Autodesk Inventor part; units mm, degrees
ref_plane "YZ Plane" through (0, 0, 0) normal (1, 0, 0) x (0, 1, 0)
ref_plane "XZ Plane" through (0, 0, 0) normal (0, 1, 0) x (-1, 0, 0)
ref_plane "XY Plane" through (0, 0, 0) normal (0, 0, 1) x (1, 0, 0)
sketch "Sketch1" plane through (0, 0, 0) normal (0, 0, 1) x (1, 0, 0)
  point P0 (0, 0)
sketch "Sketch2" plane through (0, 0, 0) normal (0, 0, 1) x (1, 0, 0)
  line L0 (-15, 20) -> (15, 20)
  line L1 (15, 20) -> (15, 0)
  line L2 (15, 0) -> (-15, 0)
  line L3 (-15, 0) -> (-15, 20)
  point P0 (0, 0)
  dimension "d0" = 30
  dimension "d1" = 20
  dimension "d2" = 20
  dimension "d3" = 15
extrude "Extrusion1" add sketch "Sketch2" along normal mid plane 20
sketch "Sketch3" plane through (0, 0, 10) normal (0, 0, 1) x (1, 0, 0)
  line L0 (-5, 45) -> (5, 45)
  line L1 (5, 45) -> (5, 20)
  line L2 (5, 20) -> (-5, 20)
  line L3 (-5, 20) -> (-5, 45)
  line L4 (15, 20) -> (-15, 20)
  point P0 (0, 0)
  dimension "d6" = 10
  dimension "d7" = 25
  dimension "d8" = 0
  dimension "d9" = 5
extrude "Extrusion2" add sketch "Sketch3" against normal blind 20
sketch "Sketch4" plane through (0, 0, 10) normal (0, 0, 1) x (1, 0, 0)
  line L0 (-15, 165) -> (15, 165)
  line L1 (15, 165) -> (15, 45)
  line L2 (15, 45) -> (-15, 45)
  line L3 (-15, 45) -> (-15, 165)
  line L4 (-5, 45) -> (5, 45)
  point P0 (0, 0)
  dimension "d12" = 30
  dimension "d13" = 120
  dimension "d14" = 0
  dimension "d15" = 15
extrude "Extrusion3" add sketch "Sketch4" against normal blind 20
sketch "Sketch5" plane through (0, 0, 10) normal (0, 0, 1) x (1, 0, 0)
  point P0 (0, 0)
sketch "Sketch6" plane through (0, 0, 10) normal (0, 0, 1) x (1, 0, 0)
  line L0 (0, 45) -> (0, 165)
  line L1 (-15, 165) -> (15, 165)
  line L2 (0, 165) -> (0, 125)
  line L3 (0, 125) -> (0, 85)
  line L4 (0, 85) -> (0, 45)
  line L5 (0, 165) -> (0, 145)
  line L6 (0, 125) -> (0, 105)
  line L7 (0, 85) -> (0, 65)
  line L8 (0, 165) -> (0, 145)
  circle A0 centre (0, 145) radius 12.5
  point P0 (0, 0)
  dimension "d18" = 40
  dimension "d19" = 40
  dimension "d20" = 20
  dimension "d21" = 20
  dimension "d22" = 20
  dimension "d23" = 25
extrude "Extrusion4" cut sketch "Sketch6" against normal blind 5
sketch "Sketch7" plane through (0, 0, 10) normal (0, 0, 1) x (1, 0, 0)
  line L0 (-15, 165) -> (15, 165)
  line L1 (0, 165) -> (0, 105)
  circle A0 centre (0, 105) radius 12.5
  point P0 (0, 0)
  dimension "d26" = 60
  dimension "d27" = 25
extrude "Extrusion5" cut sketch "Sketch7" against normal blind 5
sketch "Sketch8" plane through (0, 0, 10) normal (0, 0, 1) x (1, 0, 0)
  line L0 (0, 45) -> (0, 65)
  circle A0 centre (0, 65) radius 12.5
  point P0 (0, 0)
  dimension "d30" = 20
  dimension "d31" = 25
extrude "Extrusion6" cut sketch "Sketch8" against normal blind 5
sketch "Sketch9" plane through (15, 45, 10) normal (1, 0, 0) x (0, 0, -1)
  point P0 (10, -45)
sketch "Sketch10" plane through (0, 0, 10) normal (0, 0, 1) x (1, 0, 0)
  point P0 (0, 0)
properties part number "trafficlight"
Build history of the part. All positions in model axes, mm. A direction names the side the tool comes from. Round coordinates to 2 decimals unless told otherwise and drop trailing zeros. Loops run counter-clockwise (first coordinate to the right, second up) from the corner with the lowest first, then second, coordinate; pieces in that order, holes last. Notation, with made-up numbers: (59, 1) -> (115, 1) arc R24 cw to (115, 29) -> close; hole circle Ø5 at (72, 68). An arc over 180 degrees is marked (long way). One line per item, written item: value. Start each with the question number.
Q1. Cut at A-A on x = -11. List the corners of the cut face in (y, z).
Q2. Probe line 1 along Y through (x, z) = (0, 7.6); line 2 along X through (y, z) = (145, 6.9); line 3 along Y through (x, z) = (8.75, -6). List the from-to ranges inside material, lowest first.
Q3. Two-plate mould, pull along X, no slides. Class faces 5 (the face through (5, 33, 0)), 6 (the face through (-1.627, 157.394, 7.535)), 7 (the face through (0, 0, 0)): released by +X, released by -X, zero draft, split by the parting line, or undercut.
Q4. Cut at B-B on z = 8. List the corners of the cut face in (x, y).
Q5. Drop flat-ended pins along their axis: pin 1 Ø1.5 at (x, y) = (-5, 113.5) entering from +Z; pin 2 Ø8 at (y, z) = (29, 4) entering from +X; pin 3 Ø1.5 at (y, z) = (22, -2.5) entering from -X. Give the stop position or say it passes through.
Q6. Cut at C-C on y = 65. List the corners of the cut face in (x, z).
Q7. 3-axis set-ups, long thin cutter, end or side, ignore diameter. For faces 1 (the face through (-15, 10, 0)), 2 (the face through (10, 20, 0)), 3 (the face through (-10, 20, 0)), 4 (the face through (0, 65, 5)): which of +Z, -Z, +X, -X, +Y, -Y reach the whole face in a straight line?
Q8. Cut at D-D on x = 0. List the corners of the cut face in (y, z).
Computed:
1. outline: (0, -10) -> (20, -10) -> (20, 10) -> (0, 10) -> close; (45, -10) -> (165, -10) -> (165, 10) -> (150.94, 10) -> (150.94, 5) -> (139.06, 5) -> (139.06, 10) -> (110.94, 10) -> (110.94, 5) -> (99.06, 5) -> (99.06, 10) -> (70.94, 10) -> (70.94, 5) -> (59.06, 5) -> (59.06, 10) -> (45, 10) -> close
2. line 1: 0 to 52.5, 77.5 to 92.5, 117.5 to 132.5, 157.5 to 165
2. line 2: -15 to -12.5, 12.5 to 15
2. line 3: 0 to 20, 45 to 165
3. face 5: released by +X
3. face 6: undercut
3. face 7: zero draft
4. outline: (-15, 0) -> (15, 0) -> (15, 20) -> (5, 20) -> (5, 45) -> (15, 45) -> (15, 165) -> (-15, 165) -> (-15, 45) -> (-5, 45) -> (-5, 20) -> (-15, 20) -> close; hole circle Ø25 at (0, 65); hole circle Ø25 at (0, 105); hole circle Ø25 at (0, 145)
5. pin 1: z = 5
5. pin 2: x = 5
5. pin 3: x = -5
6. outline: (-15, -10) -> (15, -10) -> (15, 10) -> (12.5, 10) -> (12.5, 5) -> (-12.5, 5) -> (-12.5, 10) -> (-15, 10) -> close
7. face 1: +Z, -Z, -X, +Y, -Y
7. face 2: +Z, -Z, +X
7. face 3: +Z, -Z, -X
7. face 4: +Z
8. outline: (0, -10) -> (165, -10) -> (165, 10) -> (157.5, 10) -> (157.5, 5) -> (132.5, 5) -> (132.5, 10) -> (117.5, 10) -> (117.5, 5) -> (92.5, 5) -> (92.5, 10) -> (77.5, 10) -> (77.5, 5) -> (52.5, 5) -> (52.5, 10) -> (0, 10) -> close
